```python
from build123d import *

# Parameters (mm, degrees)
SKETCH1_R           = 8
SKETCH1_R_2         = 3
BOSS_EXTRUDE1_DEPTH = 2.5
FILLET2_R           = 0.3


with BuildPart() as part:
    # Sketch1 → Boss-Extrude1 (new, symmetric)
    with BuildSketch(Plane.XY):
        Circle(SKETCH1_R)
        Circle(SKETCH1_R_2, mode=Mode.SUBTRACT)
    extrude(amount=BOSS_EXTRUDE1_DEPTH, both=True)

    # Fillet2
    fillet2_edges = [part.edges().sort_by_distance(p)[0] for p in [
        (-8, 0, -2.5),
        (-8, 0, 2.5),
        (-3, 0, -2.5),
    ]]
    fillet(fillet2_edges, radius=FILLET2_R)


solid = part.part
```
The listing builds one solid part. Answer for the finished solid, in the listing's coordinates (mm). Coordinates: 2 decimals unless noted, no trailing zeros. Order: outer loops, then holes, each group sorted by start corner. A loop starts at its lowest first (then second) coordinate and runs counter-clockwise, first axis right, second up. Notation, with made-up numbers: M 63.5,54.25 L 115.5,54.25 A8 cw 115.5,58.25 Z; hole C -33.5,56 d8. An arc over 180 degrees is marked long. Answer as a JSON object with one key per item and string values. Group by question number.
1. Section A-A on y = 0 is taken. Write down the section's boundary in (x, z).
2. Straight lines are drawn through the part: line 1 (Y direction, x = 0, z = 1.5); line 2 (X direction, y = -2, z = -1.3); line 3 (X direction, y = 1.25, z = 1). For each, find the intervals that lie inside material, in ascending order.
3. Determine the mould class of faces 1 (the cylindrical face through (-3, 0, 0)), 2 (the cylindrical face through (-1.73, -7.81, 0.03)), 3 (the flat face through (3.3, 0.1, 2.5)) for opening direction Y: released by +Y, released by -Y, zero draft, split by the parting line, or undercut.
4. Flat-ended cylindrical pins translate along their axes: P1, Ø3.5, axis at x = 0, y = 0, coming from the -Z side; P2, Ø3, axis at y = -3, z = -1, coming from the +X side; P3, Ø1, axis at x = -4.5, z = 1, coming from the -Y side; P4, Ø1.5, axis at y = -5.5, z = -1, coming from the +X side. Find the tip coordinate at first contact, or state that the pin passes through.
5. Section C-C on z = -0.3 is taken. Write down the section's boundary in (x, y).
Values follow:
{
 "1": {"outline": "M -8,-2.2 A0.3 ccw -7.7,-2.5 L -3.3,-2.5 A0.3 ccw -3,-2.2 L -3,2.5 L -7.7,2.5 A0.3 ccw -8,2.2 Z; M 3,-2.2 A0.3 ccw 3.3,-2.5 L 7.7,-2.5 A0.3 ccw 8,-2.2 L 8,2.2 A0.3 ccw 7.7,2.5 L 3,2.5 Z"},
 "2": {"line 1": "-8 to -3, 3 to 8", "line 2": "-7.75 to -2.24, 2.24 to 7.75", "line 3": "-7.9 to -2.73, 2.73 to 7.9"},
 "3": {"face 1": "undercut", "face 2": "split by the parting line", "face 3": "zero draft"},
 "4": {"P1": "through", "P2": "x = 7.86", "P3": "y = -6.93", "P4": "x = 6.44"},
 "5": {"outline": "C 0,0 d16; hole C 0,0 d6"}
}
